Geometry: final body of the model. Coordinates: model frame, mm. A direction names the side the tool comes from. Give positions to 0.01 mm unless a question says otherwise; leave off trailing zeros. Write each loop counter-clockwise with the first axis right and the second up, starting at its lowest first coordinate (ties: lowest second). Pieces come first, ordered by that corner, then holes.
Q1. Line query: L1, parallel to X at y = 2.8, z = -99.5; L2, parallel to X at y = 5.75, z = -79; L3, parallel to X at y = 3.85, z = -99.5. Output: solid intervals per line, ascending.
Q2. Cut plane A-A on z = -87. Return the cut outline in (x, y), plus the area to 3 significant figures.
Q3. Cut plane D-D on x = 45. Return the cut outline in (y, z).
Q4. Cut plane C-C on y = 4.25. Count the separate pieces of the cut face and the enclosed holes in it, plus the area to 3 significant figures.
Q5. Pin query (flat end, axial travel): pin 1 (5 mm diameter, centred on x = 45, z = -99.5, fed in from +Y); pin 2 (4 mm diameter, centred on x = 108.5, z = -3.5, fed in from -Y). Return the tip coordinate at first contact, or that it passes through.
Q6. Cut plane B-B on x = 135. Return the cut outline in (y, z), plus the area to 3 significant figures.
Q7. Reachability of faces 1 (the face through (218, 3, -51)), 2 (the face through (9, 3, -53)), 3 (the face through (107.874, 1.479, -95.923)) from +Z, -Z, +X, -X, +Y, -Y: full face, straight path, thin tool, end or side. Return the list, or none.
```python
from build123d import *

# Parameters (mm, degrees)
BOSS_EXTRUDE1_DEPTH = 7
FILLET1_R           = 5
SKETCH2_R           = 2
CUT_EXTRUDE1_DEPTH  = 121.971070922
SKETCH3_R           = 3.75
CUT_EXTRUDE2_DEPTH  = 3
CHAMFER1_SIZE       = 1


with BuildPart() as part:
    # Sketch1 → Boss-Extrude1 (new body)
    with BuildSketch(Plane(origin=(0, 0, 0), x_dir=(1, 0, 0), z_dir=(0, 1, 0))):
        with BuildLine():
            Line((0, 0), (109, 0))
            Line((109, 0), (109, 34))
            ThreePointArc((109, 34), (104.050252532, 36.050252532), (102, 41))
            Line((102, 41), (102, 52))
            Line((102, 52), (85, 52))
            Line((85, 52), (85, 9))
            Line((85, 9), (9, 9))
            Line((9, 9), (9, 52))
            Line((9, 52), (0, 52))
            Line((0, 52), (0, 0))
        make_face()
    extrude(amount=BOSS_EXTRUDE1_DEPTH)

    # Fillet1
    fillet1_edges = [part.edges().sort_by_distance(p)[0] for p in [
        (9, 3.5, -9),
        (85, 3.5, -9),
    ]]
    fillet(fillet1_edges, radius=FILLET1_R)

    # Sketch2 → Cut-Extrude1 (cut, through all)
    with BuildSketch(Plane(origin=(0, 7, 0), x_dir=(1, 0, 0), z_dir=(0, 1, 0))):
        with Locations(Location((5, 4.5, 0), (0, 0, 270))):
            Circle(SKETCH2_R)
        with Locations(Location((45, 4.5, 0), (0, 0, 270))):
            Circle(SKETCH2_R)
    extrude(amount=-CUT_EXTRUDE1_DEPTH, mode=Mode.SUBTRACT)

    # Sketch3 → Cut-Extrude2 (cut)
    with BuildSketch(Plane(origin=(0, 0, 0), x_dir=(-1, 0, 0), z_dir=(0, -1, 0))):
        with Locations((-109, 4.5)):
            Circle(SKETCH3_R)
    extrude(amount=-CUT_EXTRUDE2_DEPTH, mode=Mode.SUBTRACT)

    # Chamfer1
    chamfer1_edges = [part.edges().sort_by_distance(p)[0] for p in [
        (5, 7, -6.5),
        (45, 7, -6.5),
    ]]
    chamfer(chamfer1_edges, length=CHAMFER1_SIZE)

    # Mirror1: part across plane


with BuildPart() as part_1:
    add(part.part)
    add(part.part.mirror(Plane(origin=(9, 7, -52), x_dir=(1, 0, 0), z_dir=(0, 0, 1))))

    # Mirror2: part across plane


with BuildPart() as part_2:
    add(part_1.part)
    add(part_1.part.mirror(Plane(origin=(109, 7, -104), x_dir=(0, 0, 1), z_dir=(-1, 0, 0))))


solid = part_2.part
```
Data:
1. L1: x = 0 to 3, 7 to 43, 47 to 105.25, 112.75 to 171, 175 to 211, 215 to 218
1. L2: x = 0 to 9, 85 to 133, 209 to 218
1. L3: x = 0 to 3, 7 to 43, 47 to 171, 175 to 211, 215 to 218
2. outline: (0, 0) - (9, 0) - (9, 7) - (0, 7) - close; (85, 0) - (133, 0) - (133, 7) - (85, 7) - close; (209, 0) - (218, 0) - (218, 7) - (209, 7) - close
2. area: 462 mm2
3. outline: (0, -104) - (7, -104) - (7, -102.5) - (6, -101.5) - (0, -101.5) - close; (0, -97.5) - (6, -97.5) - (7, -96.5) - (7, -95) - (0, -95) - close; (0, -9) - (7, -9) - (7, -7.5) - (6, -6.5) - (0, -6.5) - close; (0, -2.5) - (6, -2.5) - (7, -1.5) - (7, 0) - (0, 0) - close
4. separate pieces: 1
4. enclosed holes: 11
4. area: 9,080 mm2
5. pin 1: stops at y = 6.5
5. pin 2: stops at y = 3
6. outline: (0, -104) - (7, -104) - (7, -94) - (0, -94) - close; (0, -10) - (7, -10) - (7, 0) - (0, 0) - close
6. area: 140 mm2
7. face 1: +Z, -Z, +X, +Y, -Y
7. face 2: +Y, -Y
7. face 3: -Y
